Source: CAD feature listing. Evaluate the final solid. Frame: model axes, mm. Coordinates: 2 decimals unless noted, no trailing zeros. Write each loop counter-clockwise with the first axis right and the second up, starting at its lowest first coordinate (ties: lowest second). Pieces come first, ordered by that corner, then holes. Notation, with made-up numbers: M -10.75,76.25 L 28.25,76.25 A24 ccw 28.25,99.25 Z; hole C -24,-28.75 d2. An arc over 180 degrees is marked long. Write item = value, one per line. Start each with the question number.
1. Pin query (flat end, axial travel): pin 1 Ø1.4 at (x, y) = (-9, -1) entering from +Z; pin 2 Ø0.5 at (x, y) = (4.5, -1.5) entering from +Z; pin 3 Ø0.9 at (x, y) = (-7.5, -0.5) entering from -Z. Return the tip coordinate at first contact, or that it passes through.
2. Section query C-C (x = 6). Output: boundary loops of the cut face in (y, z), then the cut area to 3 significant figures.
3. Section query A-A (x = -8.5). Output: boundary loops of the cut face in (y, z).
4. Line query: line 1 along Z through (x, y) = (12, -1.05); line 2 along Z through (x, y) = (-6, -0.5); line 3 along X through (y, z) = (-1.9, -3.5). Output: solid intervals per line, ascending.
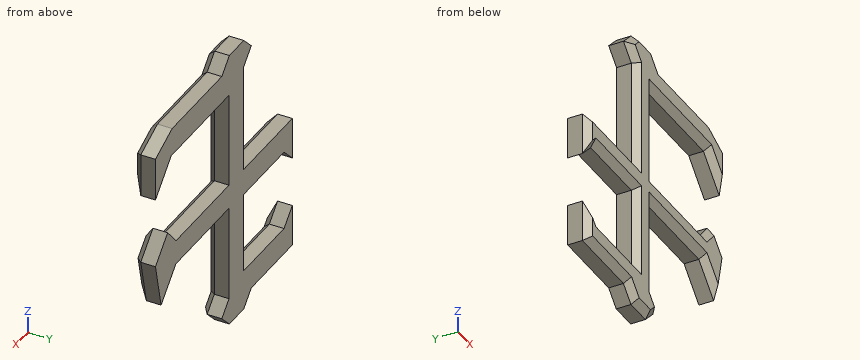
```python
from build123d import *

# Parameters (mm, degrees)
F1_DEPTH = 5.08
F2_SIZE  = 1.5875
F3_SCALE = 0.5


with BuildPart() as f1:
    # F0 (on Front) → F1 (new body)
    with BuildSketch(Plane.XZ):
        Polygon((-6.6455395231, 29.4341069916), (-3.175, 25.9635674685), (-3.175, 0.1128360473), (-24.7444733058, 0.1128360473), (-24.7444733058, -9.883693457), (-21.0979438016, -6.2371639527), (-3.175, -6.2371639527), (-3.175, -25.5762760587), (-21.0979438016, -25.5762760587), (-24.7444733058, -21.9297465545), (-24.7444733058, -31.9262760587), (-22.1278171024, -31.9262760587), (-6.6455395231, -31.9262760587), (-3.3227697615, -35.2490458202), (3.0272302385, -35.2490458202), (6.35, -31.9262760587), (3.175, -28.7512760587), (3.175, -5.8234985377), (26.6026397626, -5.8234985377), (33.1378690898, -12.3587278649), (35.6206595898, -1.1474714229), (30.2332143891, 4.2399737777), (26.6026397626, 0), (3.175, 0), (3.175, 22.7885674685), (28.6609344184, 22.7885674685), (35.6206595898, 15.7537590712), (35.6206595898, 26.0716768982), (28.2596744327, 29.4341069916), (6.35, 29.4341069916), (3.0272302385, 32.7568767531), (-3.3227697615, 32.7568767531), align=None)
    extrude(amount=F1_DEPTH)

    # F2
    f2_edges = [f1.edges().sort_by_distance(p)[0] for p in [
        (17.304837, -5.08, 29.434107),
        (4.688615, -5.08, 31.095492),
        (-0.14777, -5.08, 32.756877),
        (-4.984155, -5.08, 31.095492),
        (-4.91027, -5.08, 27.698837),
        (-3.175, -5.08, 13.038202),
        (-13.959737, -5.08, 0.112836),
        (-24.744473, -5.08, -4.885429),
        (-22.921209, -5.08, -8.060429),
        (-12.136472, -5.08, -6.237164),
        (-3.175, -5.08, -15.90672),
        (-12.136472, -5.08, -25.576276),
        (-22.921209, -5.08, -23.753011),
        (-24.744473, -5.08, -26.928011),
        (-15.695006, -5.08, -31.926276),
        (-4.984155, -5.08, -33.587661),
        (-0.14777, -5.08, -35.249046),
        (4.688615, -5.08, -33.587661),
        (4.7625, -5.08, -30.338776),
        (3.175, -5.08, -17.287387),
        (14.88882, -5.08, -5.823499),
        (29.870254, -5.08, -9.091113),
        (34.379264, -5.08, -6.7531),
        (32.926937, -5.08, 1.546251),
        (28.417927, -5.08, 2.119987),
        (14.88882, -5.08, 0),
        (3.175, -5.08, 11.394284),
        (15.917967, -5.08, 22.788567),
        (32.140797, -5.08, 19.271163),
        (35.62066, -5.08, 20.912718),
        (31.940167, -5.08, 27.752892),
    ]]
    chamfer(f2_edges, length=F2_SIZE)


with BuildPart() as f1_1:
    # F3: moved
    add(f1.part.scale(F3_SCALE))


solid = f1_1.part
```
Results are:
q1.pin_1 = 0.06
q1.pin_2 = 14.72
q1.pin_3 = -15.96
q2.outline = M -2.54,-2.12 L -1.75,-2.91 L 0,-2.91 L 0,0 L -1.75,0 L -2.54,-0.79 Z; M -2.54,12.19 L -1.75,11.39 L 0,11.39 L 0,14.72 L -1.75,14.72 L -2.54,13.92 Z
q2.area = 14.6 mm^2
q3.outline = M -2.54,-15.17 L -1.75,-15.96 L 0,-15.96 L 0,-12.79 L -1.75,-12.79 L -2.54,-13.58 Z; M -2.54,-2.32 L -1.75,-3.12 L 0,-3.12 L 0,0.06 L -1.75,0.06 L -2.54,-0.74 Z
q4.line_1 = -2.91 to 0, 11.39 to 14.72
q4.line_2 = -15.96 to -12.79, -3.12 to 0.06
q4.line_3 = -12.22 to -11.15, -1.43 to 1.43, 14.11 to 17
